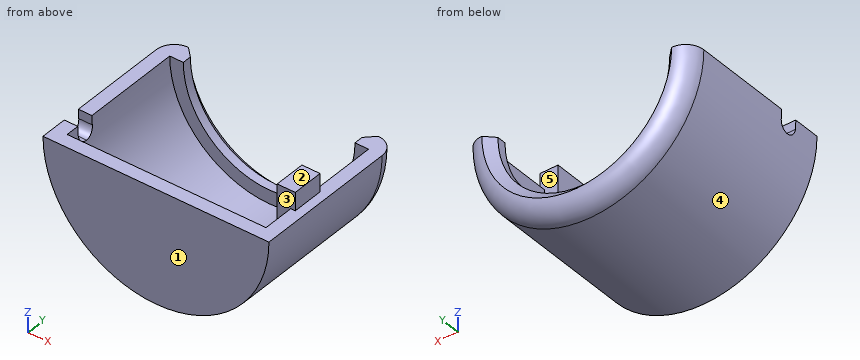
```python
from build123d import *

# Parameters (mm, degrees)
R_VOLUTION1_ANGLE              = 180
CHANFREIN1_SIZE                = 1
CONG_1_R                       = 2
ENL_V_MAT_EXTRU_1_REACH        = 27.229
ESQUISSE4_W                    = 4
ESQUISSE4_H                    = 2
CONG_2_R                       = 1
BOSS_EXTRU_2_REACH             = 27.229
BOSS_EXTRU_2_END_RADIUS        = 11
ESQUISSE5_W                    = 2
ESQUISSE5_H                    = 3.5
BOSS_EXTRU_2_DIRECTION_2_DEPTH = 2


with BuildPart() as part:
    # Esquisse3 → Révolution1 (revolve)
    with BuildSketch(Plane.XY):
        Polygon((0, 0), (12.5, 0), (12.5, 18), (9.5, 18), (9.5, 16), (11, 16), (11, 1.5), (0, 1.5), align=None)
    revolve(axis=Axis((0, 0, 0), (0, 1, 0)), revolution_arc=R_VOLUTION1_ANGLE)

    # Chanfrein1
    chanfrein1_edges = [part.edges().sort_by_distance(p)[0] for p in [
        (0, 18, -9.5),
    ]]
    chamfer(chanfrein1_edges, length=CHANFREIN1_SIZE)

    # Congé1
    cong_1_edges = [part.edges().sort_by_distance(p)[0] for p in [
        (0, 18, -12.5),
    ]]
    fillet(cong_1_edges, radius=CONG_1_R - 0.0001)  # a hair under: the kernel refuses the full size

    # Esquisse4 → Enlèv. mat.-Extru.1 (cut, up to next)
    with BuildSketch(Plane(origin=(0, 0, 0), x_dir=(0, 0, -1), z_dir=(1, 0, 0)), mode=Mode.PRIVATE) as enl_v_mat_extru_1_sk1:
        with Locations((0, 4)):
            Rectangle(ESQUISSE4_W, ESQUISSE4_H)
    enl_v_mat_extru_1_tool1 = extrude(enl_v_mat_extru_1_sk1.sketch, amount=-ENL_V_MAT_EXTRU_1_REACH, mode=Mode.PRIVATE) & part.part
    add(enl_v_mat_extru_1_tool1.solids().sort_by_distance((0, 4, 0))[0], mode=Mode.SUBTRACT)

    # Congé2
    cong_2_edges = [part.edges().sort_by_distance(p)[0] for p in [
        (-11.577808253, 5, -2),
        (-11.577808253, 3, -2),
    ]]
    fillet(cong_2_edges, radius=CONG_2_R - 0.0001)  # a hair under: the kernel refuses the full size

    # Boss.-Extru.2: up to this cylinder (the profile starts inside it)
    boss_extru_2_end = Plane(origin=(0, 6.75, 0), z_dir=(0, -1, 0)) * Cylinder(BOSS_EXTRU_2_END_RADIUS, 77.458, mode=Mode.PRIVATE)
    # Esquisse5 → Boss.-Extru.2 (add, up to the surface)
    with BuildSketch(Plane.XY, mode=Mode.PRIVATE) as boss_extru_2_sk1:
        with Locations((10.5, 6.75)):
            Rectangle(ESQUISSE5_W, ESQUISSE5_H)
    boss_extru_2_tool1 = extrude(boss_extru_2_sk1.sketch, amount=-BOSS_EXTRU_2_REACH, mode=Mode.PRIVATE) & boss_extru_2_end
    add(boss_extru_2_tool1.solids().sort_by_distance((10.5, 6.75, 0))[0])

    # Esquisse5 → Boss.-Extru.2 direction 2 (add)
    with BuildSketch(Plane.XY):
        with Locations((10.5, 6.75)):
            Rectangle(ESQUISSE5_W, ESQUISSE5_H)
    extrude(amount=BOSS_EXTRU_2_DIRECTION_2_DEPTH)


solid = part.part
```
Geometry check sheet. Reference: the model listing, model coordinates, mm. Face numbers are marked on the shaded views. A direction names the side the tool comes from. Coordinates: 2 decimals unless noted, no trailing zeros. Write each loop counter-clockwise with the first axis right and the second up, starting at its lowest first coordinate (ties: lowest second). Pieces come first, ordered by that corner, then holes. Notation, with made-up numbers: (65.25, 75.25) -> (116.25, 75.25) arc R17 cw to (116.25, 84.25) -> close; hole circle Ø4 at (37, 38.5). An arc over 180 degrees is marked (long way). Use CSV: the item, a comma, the result in double quotes. Start each with the question number.
Item 1: Mould release check, pull along Y, two halves, no side actions. Record for the marked faces 1, 2 and 3: released by +Y, released by -Y, zero draft, split by the parting line, or undercut.
Item 2: Depth check by flat-ended pin: pin 1 Ø3 at (x, y) = (-7.5, 13) entering from +Z; pin 2 Ø5.5 at (x, y) = (2, 13) entering from +Z; pin 3 Ø3 at (x, z) = (9, -8.5) entering from +Y. Enter the tip coordinate at first touch or a pass-through.
Item 3: Cross-section at A-A, the plane y = 7. Record the cut outline in (x, z), plus the area to 3 significant figures.
Item 4: Thickness scan on line 1 (Y direction, x = -1.75, z = -8.5); line 2 (Y direction, x = -2.75, z = -10.5); line 3 (Z direction, x = 1, y = 11.5). Record the ranges inside material, lowest first.
Item 5: Set-up check for the marked faces 4 and 5: record each of +Z, -Z, +X, -X, +Y, -Y from which the full face is reachable in a straight line by a thin tool's end or side.
Item 6: Cross-section at B-B, the plane y = 15. Record the cut outline in (x, z), plus the area to 3 significant figures.
Answers:
1,face 1,"released by -Y"
1,face 2,"zero draft"
1,face 3,"undercut"
2,pin 1,"z = -6.32"
2,pin 2,"z = -9.92"
2,pin 3,"y = 17.96"
3,outline,"(-12.5, 0) arc R12.5 ccw to (12.5, 0) -> (11.5, 0) -> (11.5, 2) -> (9.5, 2) -> (9.5, -5.55) arc R11 cw to (-11, 0) -> close"
3,area,"65.0 mm^2"
4,line 1,"0 to 1.5"
4,line 2,"0 to 1.5, 16 to 17.97"
4,line 3,"-12.46 to -10.95"
5,face 4,"-Z, +Y, -Y"
5,face 5,"+Z"
6,outline,"(-12.5, 0) arc R12.5 ccw to (12.5, 0) -> (11, 0) arc R11 cw to (-11, 0) -> close"
6,area,"55.4 mm^2"
